Verification items for the finished model (mm, model axes). A direction names the side the tool comes from. Give positions to 0.01 mm unless a question says otherwise; leave off trailing zeros. Write each loop counter-clockwise with the first axis right and the second up, starting at its lowest first coordinate (ties: lowest second). Pieces come first, ordered by that corner, then holes.
from build123d import *

# Parameters (mm, degrees)
SKETCH_R     = 75
PAD_DEPTH    = 210
FILLET_R     = 45
FILLET001_R  = 20
SKETCH001_R  = 40
PAD001_DEPTH = 15
SKETCH002_R  = 42.5
PAD002_DEPTH = 10
FILLET002_R  = 2


with BuildPart() as part:
    # Sketch → Pad (new body)
    with BuildSketch(Plane.XY):
        Circle(SKETCH_R)
    extrude(amount=PAD_DEPTH)

    # Fillet
    fillet_edges = [part.edges().sort_by_distance(p)[0] for p in [
        (-75, 0, 210),
    ]]
    fillet(fillet_edges, radius=FILLET_R)

    # Fillet001
    fillet001_edges = [part.edges().sort_by_distance(p)[0] for p in [
        (-75, 0, 0),
    ]]
    fillet(fillet001_edges, radius=FILLET001_R)

    # Sketch001 (on Face5 of Fillet001) → Pad001 (join)
    with BuildSketch(Plane.XY.offset(210)):
        Circle(SKETCH001_R)
    extrude(amount=PAD001_DEPTH)

    # Sketch002 (on Face3 of Pad001) → Pad002 (join)
    with BuildSketch(Plane.XY.offset(225)):
        Circle(SKETCH002_R)
    extrude(amount=PAD002_DEPTH)

    # Fillet002
    fillet002_edges = [part.edges().sort_by_distance(p)[0] for p in [
        (-42.5, 0, 235),
    ]]
    fillet(fillet002_edges, radius=FILLET002_R)


solid = part.part
Item 1: Sectioned sample at A-A on z = 88. Record the cut outline in (x, y), then the cut area to 3 significant figures.
Answer key:
outline: circle Ø150 at (0, 0)
area: 17,700 mm2
Item 2: Set-up check for faces 1 (the face through (-9.764, 74.362, 91.485)), 2 (the face through (-29, -28, 225)): record each of +Z, -Z, +X, -X, +Y, -Y from which the full face is reachable in a straight line by a thin tool's end or side.
Answer key:
face 1: +Z, -Z
face 2: none
Item 3: Scan lines: line 1 along Z through (x, y) = (37, 3); line 2 along Z through (x, y) = (-37.5, -13); line 3 along Z through (x, y) = (9, -48.5). Record each from-to range of solid material in increasing order.
Answer key:
line 1: z = 0 to 209.43, 210 to 235
line 2: z = 0 to 208.94, 210 to 235
line 3: z = 0 to 205.64
Item 4: Release check for a two-part mould opening along Z. For faces 3 (the face through (-8.67, -39.05, 217.4)), 4 (the face through (-33.727, -25.861, 228.944)), 5 (the face through (-1, 1, 235)) record: released by +Z, released by -Z, zero draft, split by the parting line, or undercut.
Answer key:
face 3: undercut
face 4: zero draft
face 5: released by +Z
Item 5: Depth check by flat-ended pin: pin 1 (3 mm diameter, centred on x = 37, z = 97, fed in from +Y); pin 2 (3 mm diameter, centred on x = -56.5, y = -44.5, fed in from +Z); pin 3 (12 mm diameter, centred on x = 24, z = 175, fed in from +Y). Enter the tip coordinate at first touch or a pass-through.
Answer key:
pin 1: stops at y = 66.07
pin 2: stops at z = 184.78
pin 3: stops at y = 72.04
